Source: CAD feature listing. Evaluate the final solid. Frame: model axes, mm. A direction names the side the tool comes from. Give positions to 0.01 mm unless a question says otherwise; leave off trailing zeros. Loops run counter-clockwise (first coordinate to the right, second up) from the corner with the lowest first, then second, coordinate; pieces in that order, holes last. Notation, with made-up numbers: (75.5, -22.75) -> (92.5, -22.75) arc R33 cw to (92.5, 5.25) -> close; hole circle Ø9 at (34.5, -40). An arc over 180 degrees is marked (long way). Return JSON: item names as keys, results as strings. Group by question number.
(1) Ray query, line 1 (Z direction, x = 1.6, y = 2.5); line 2 (Z direction, x = 3.35, y = 14); line 3 (Y direction, x = 2.05, z = 11.5). Return the intervals inside material, ascending. Write a range as from..to.
(2) Cut plane C-C on y = 26. Return loops of the section in (x, z), then the cut area to 3 significant figures.
(3) Cut plane A-A on y = 3. Return loops of the section in (x, z).
(4) Cut plane B-B on x = 3.4. Return loops of the section in (y, z), then the cut area to 3 significant figures.
(5) Pin query (flat end, axial travel): pin 1 (1.2 mm diameter, centred on x = 2.5, y = 2, fed in from +Z); pin 2 (1 mm diameter, centred on x = 3, y = 7.5, fed in from +Z). Return the tip coordinate at first contact, or that it passes through.
(6) Draft query along Z for faces 1 (the face through (2, 0, 10)), 2 (the face through (2, 19, 10)), 3 (the face through (2, 4, 6)), 4 (the face through (2, 2, 8)). Return one class per face: released by +Z, released by -Z, zero draft, split by the parting line, or undercut.
(7) Cut plane D-D on z = 14. Return loops of the section in (x, y).
(8) Access query for faces 5 (the face through (2, 4, 14)), 6 (the face through (2, 2, 4)), 7 (the face through (2, 0, 2)). Directions: +Z, -Z, +X, -X, +Y, -Y. A direction counts if a zero-diameter tool reaches every point of the face in a straight line with its end or side. Return the directions, or none.
```python
from build123d import *

# Parameters (mm, degrees)
F0_W     = 4
F0_H     = 4
F1_DEPTH = 4


with BuildPart() as f1:
    # F0 (on Right) → F1 (new body)
    with BuildSketch(Plane.YZ):
        with BuildLine():
            Line((4, 4), (4, 0))
            Line((4, 0), (33.614835, 0))
            ThreePointArc((33.614835, 0), (35.578748, 1.621785), (34.357617, 3.856953))
            Line((34.357617, 3.856953), (4, 16))
            Line((4, 16), (4, 12))
            Line((4, 12), (4, 8))
            Line((4, 8), (4, 4))
        make_face()
        with Locations((2, 10)):
            Rectangle(F0_W, F0_H)
        with Locations((2, 2)):
            Rectangle(F0_W, F0_H)
    extrude(amount=F1_DEPTH)


solid = f1.part
```
Answers:
{
 "1": {"line 1": "0..4, 8..12", "line 2": "0..12", "line 3": "0..15.25"},
 "2": {"outline": "(0, 0) -> (4, 0) -> (4, 7.2) -> (0, 7.2) -> close", "area": "28.8 mm²"},
 "3": {"outline": "(0, 0) -> (4, 0) -> (4, 4) -> (0, 4) -> close; (0, 8) -> (4, 8) -> (4, 12) -> (0, 12) -> close"},
 "4": {"outline": "(0, 0) -> (33.61, 0) arc R2 ccw to (34.36, 3.86) -> (4, 16) -> (4, 12) -> (0, 12) -> (0, 8) -> (4, 8) -> (4, 4) -> (0, 4) -> close", "area": "337 mm²"},
 "5": {"pin 1": "z = 12", "pin 2": "z = 14.8"},
 "6": {"face 1": "zero draft", "face 2": "released by +Z", "face 3": "undercut", "face 4": "undercut"},
 "7": {"outline": "(0, 4) -> (4, 4) -> (4, 9) -> (0, 9) -> close"},
 "8": {"face 5": "+Z, +X, -X, -Y", "face 6": "+X, -X, -Y", "face 7": "+Z, -Z, +X, -X, -Y"}
}
